from build123d import *

# Parameters (mm, degrees)
BOSS_EXTRUDE1_DEPTH = 4
SKETCH2_R           = 23
BOSS_EXTRUDE2_DEPTH = 4
SKETCH3_R           = 45
BOSS_EXTRUDE3_DEPTH = 6
SKETCH4_R           = 40
SKETCH4_R_2         = 19
CUT_EXTRUDE1_DEPTH  = 6
SKETCH5_R           = 14
CUT_EXTRUDE2_DEPTH  = 8
SKETCH6_R           = 7
CUT_EXTRUDE3_DEPTH  = 81.888663881
FILLET1_R           = 2
SKETCH7_R           = 3.5
CUT_EXTRUDE4_DEPTH  = 82.110886719


with BuildPart() as part:
    # Sketch1 → Boss-Extrude1 (new body)
    with BuildSketch(Plane(origin=(0, 0, 0), x_dir=(1, 0, 0), z_dir=(0, 1, 0))):
        with BuildLine():
            Line((2, -60.044427996), (51, -31.754264805))
            ThreePointArc((51, -31.754264805), (52.464101615, -30.29016319), (53, -28.29016319))
            Line((53, -28.29016319), (53, 28.29016319))
            ThreePointArc((53, 28.29016319), (52.464101615, 30.29016319), (51, 31.754264805))
            Line((51, 31.754264805), (2, 60.044427996))
            ThreePointArc((2, 60.044427996), (0, 60.580326381), (-2, 60.044427996))
            Line((-2, 60.044427996), (-51, 31.754264805))
            ThreePointArc((-51, 31.754264805), (-52.464101615, 30.29016319), (-53, 28.29016319))
            Line((-53, 28.29016319), (-53, -28.29016319))
            ThreePointArc((-53, -28.29016319), (-52.464101615, -30.29016319), (-51, -31.754264805))
            Line((-51, -31.754264805), (-2, -60.044427996))
            ThreePointArc((-2, -60.044427996), (0, -60.580326381), (2, -60.044427996))
        make_face()
    extrude(amount=BOSS_EXTRUDE1_DEPTH)

    # Sketch2 → Boss-Extrude2 (add)
    with BuildSketch(Plane(origin=(0, 4, 0), x_dir=(1, 0, 0), z_dir=(0, 1, 0))):
        with Locations(Location((0, 0, 0), (0, 0, 270))):
            Circle(SKETCH2_R)
    extrude(amount=BOSS_EXTRUDE2_DEPTH)

    # Sketch3 → Boss-Extrude3 (add)
    with BuildSketch(Plane.XZ):
        with Locations(Location((0, 0, 0), (0, 0, 270))):
            Circle(SKETCH3_R)
    extrude(amount=BOSS_EXTRUDE3_DEPTH)

    # Sketch4 → Cut-Extrude1 (cut)
    with BuildSketch(Plane.XZ.offset(6)):
        with Locations(Location((0, 0, 0), (0, 0, 270))):
            Circle(SKETCH4_R)
        with Locations(Location((0, 0, 0), (0, 0, 270))):
            Circle(SKETCH4_R_2, mode=Mode.SUBTRACT)
    extrude(amount=-CUT_EXTRUDE1_DEPTH, mode=Mode.SUBTRACT)

    # Sketch5 → Cut-Extrude2 (cut)
    with BuildSketch(Plane.XZ.offset(6)):
        with Locations(Location((0, 0, 0), (0, 0, 270))):
            Circle(SKETCH5_R)
    extrude(amount=-CUT_EXTRUDE2_DEPTH, mode=Mode.SUBTRACT)

    # Sketch6 → Cut-Extrude3 (cut, through all)
    with BuildSketch(Plane.XZ.offset(-2)):
        with Locations(Location((0, 0, 0), (0, 0, 270))):
            Circle(SKETCH6_R)
    extrude(amount=-CUT_EXTRUDE3_DEPTH, mode=Mode.SUBTRACT)

    # Fillet1
    fillet1_edges = [part.edges().sort_by_distance(p)[0] for p in [
        (0, 8, -23),
        (0, 0, 45),
        (0, -6, 19),
    ]]
    fillet(fillet1_edges, radius=FILLET1_R)

    # Sketch7 → Cut-Extrude4 (cut, through all)
    with BuildSketch(Plane(origin=(0, 4, 0), x_dir=(1, 0, 0), z_dir=(0, 1, 0))):
        with Locations(Location((0, 51, 0), (0, 0, 270))):
            Circle(SKETCH7_R)
        with Locations(Location((44.167295593, 25.5, 0), (0, 0, 270))):
            Circle(SKETCH7_R)
        with Locations(Location((44.167295593, -25.5, 0), (0, 0, 270))):
            Circle(SKETCH7_R)
        with Locations(Location((0, -51, 0), (0, 0, 270))):
            Circle(SKETCH7_R)
        with Locations(Location((-44.167295593, -25.5, 0), (0, 0, 270))):
            Circle(SKETCH7_R)
        with Locations(Location((-44.167295593, 25.5, 0), (0, 0, 270))):
            Circle(SKETCH7_R)
    extrude(amount=-CUT_EXTRUDE4_DEPTH, mode=Mode.SUBTRACT)


solid = part.part
Source: CAD feature listing. Evaluate the final solid. Frame: model axes, mm. A direction names the side the tool comes from. Give positions to 0.01 mm unless a question says otherwise; leave off trailing zeros. Write each loop counter-clockwise with the first axis right and the second up, starting at its lowest first coordinate (ties: lowest second). Pieces come first, ordered by that corner, then holes. Notation, with made-up numbers: (76.5, 66) - (99.5, 66) arc R27 ccw to (99.5, 96) - close; hole circle Ø6 at (20, 11.25). An arc over 180 degrees is marked (long way). Write item = value, one per line. Start each with the question number.
Q1. Material intervals for probe 1 along X at (y, z) = (-2.5, 0); probe 2 along X at (y, z) = (2.3, -25.5); probe 3 along X at (y, z) = (-0.75, -2), sorted ascending.
Q2. Cut plane C-C, the plane z = 51. Return loops of the section in (x, y), then the cut area to 3 significant figures.
Q3. Pin query (flat end, axial travel): pin 1 Ø1.5 at (y, z) = (1.5, 30) entering from -X; pin 2 Ø11 at (x, z) = (-44.17, -25.5) entering from -Y; pin 3 Ø8 at (x, z) = (15, -17.5) entering from +Y; pin 4 Ø16 at (x, z) = (0, 0) entering from -Y. Return the tip coordinate at first contact, or that it passes through.
Q4. Draft query along Z for faces 4 (the cylindrical face through (-39.05, -3.04, 8.67)), 5 (the flat face through (0, 8, 9)), 6 (the cylindrical face through (52.449, 1.972, 30.316)). Return one class per face: +Z half, -Z half, draft (parallel to the pull), parting line (faces both ways), or undercut.
Q5. Cut plane B-B, the plane x = 0. Give the number of separate pieces and of enclosed holes in the cut face, then the cut area to 3 significant figures.
Q6. Reachability of faces 1 (the flat face through (3.3, 2, 6.4)), 2 (the cylindrical face through (19.394, 4.986, 12.365)), 3 (the cylindrical face through (-47.27, 2.03, -23.88)) from +Z, -Z, +X, -X, +Y, -Y: full face, straight path, thin tool, end or side. Return the list, or none.
Computed values:
q1.probe_1 = -45 to -40, -19 to -14, 14 to 19, 40 to 45
q1.probe_2 = -53 to -47.67, -40.67 to 40.67, 47.67 to 53
q1.probe_3 = -45.39 to -39.95, -18.89 to -13.86, 13.86 to 18.89, 39.95 to 45.39
q2.outline = (-17.67, 0) - (-3.5, 0) - (-3.5, 4) - (-17.67, 4) - close; (3.5, 0) - (17.67, 0) - (17.67, 4) - (3.5, 4) - close
q2.area = 113 mm²
q3.pin_1 = -52.88
q3.pin_2 = -0.67
q3.pin_3 = 8
q3.pin_4 = 2
q4.face_4 = undercut
q4.face_5 = draft
q4.face_6 = +Z half
q5.separate_pieces = 4
q5.enclosed_holes = 0
q5.area = 591 mm²
q6.face_1 = -Y
q6.face_2 = +Y
q6.face_3 = +Y, -Y
